Geometry check sheet. Reference: the model listing, model coordinates, mm. A direction names the side the tool comes from. Round coordinates to 2 decimals unless told otherwise and drop trailing zeros. Order: outer loops, then holes, each group sorted by start corner. A loop starts at its lowest first (then second) coordinate and runs counter-clockwise, first axis right, second up. Notation, with made-up numbers: (-0.75, 11.5) - (34.25, 11.5) arc R26 cw to (34.25, 32.5) - close; hole circle Ø2 at (60.25, 44.5). An arc over 180 degrees is marked (long way). Return JSON: item names as keys, results as strings. Group by question number.
Q1. Gauge pin test, flat ends, axial feed: pin 1 Ø6 at (x, z) = (16, 0.5) entering from +Y; pin 2 Ø1.5 at (y, z) = (5.5, 5) entering from +X. Record the tip position at first contact, or that the pin passes through.
Q2. Sectioned sample at B-B, the plane z = -1. Record the cut outline in (x, y) (3 decimals).
Q3. Tool access check on faces 1 (the flat face through (13, 3.303, 0)), 2 (the flat face through (2, 22.215, 0)). Record the directions out of +Z, -Z, +X, -X, +Y, -Y that give a thin tool (end or side, any length) a straight path to the whole face; none if there is none.
Q4. Sectioned sample at A-A, the plane y = 4. Record the cut outline in (x, z).
Q5. Material ranges on line 1 along Y through (x, z) = (16.5, -7.25); line 2 along X through (y, z) = (7.25, -0.75), recorded low to high.
Q6. Sectioned sample at C-C, the plane x = 9. Record the cut outline in (y, z), then the cut area to 3 significant figures.
Autodesk Inventor part; units mm, degrees
sketch "Sketch1" plane through (0, 0, 0) normal (0, 0, 1) x (1, 0, 0)
  line L0 (0, 22.215) -> (0, 0)
  line L1 (0, 0) -> (22.6684, 0)
  line L2 (22.6684, 0) -> (22.6684, 3.3031)
  line L3 (22.6684, 3.3031) -> (3.2383, 3.3031)
  line L4 (3.2383, 3.3031) -> (3.2383, 22.215)
  line L5 (3.2383, 22.215) -> (0, 22.215)
  line L6 (0, 28.8795) -> (0, -2.2215)
  line L7 (-2.2668, 0) -> (29.4689, 0)
extrude "Extrusion1" add sketch "Sketch1" along normal mid plane 25.4
properties part number "solid_base_feature"
Reply:
{
 "1": {"pin 1": "y = 3.3", "pin 2": "x = 3.24"},
 "2": {"outline": "(0, 0) - (22.668, 0) - (22.668, 3.303) - (3.238, 3.303) - (3.238, 22.215) - (0, 22.215) - close"},
 "3": {"face 1": "+Z, -Z, +X, +Y", "face 2": "+Z, -Z, +X, -X, +Y"},
 "4": {"outline": "(0, -12.7) - (3.24, -12.7) - (3.24, 12.7) - (0, 12.7) - close"},
 "5": {"line 1": "0 to 3.3", "line 2": "0 to 3.24"},
 "6": {"outline": "(0, -12.7) - (3.3, -12.7) - (3.3, 12.7) - (0, 12.7) - close", "area": "83.9 mm^2"}
}
